The figure shows three views and two pictorial views of one solid part (mm, origin at its lowest corner). Answer the questions. A direction names the side the tool comes from. Round coordinates to 2 decimals unless told otherwise and drop trailing zeros. Order: outer loops, then holes, each group sorted by start corner. A loop starts at its lowest first (then second) coordinate and runs counter-clockwise, first axis right, second up. Notation, with made-up numbers: (4, 76.25) - (60, 76.25) arc R28 ccw to (60, 102.25) - close; hole circle Ø9 at (15.25, -18.5). An arc over 180 degrees is marked (long way). Use CSV: the item, a comma, the result in double quotes. Start each with the question number.
Item 1: Straight lines are drawn through the part: line 1 along Z through (x, y) = (62, 37); line 2 along X through (y, z) = (27.5, 6); line 3 along Z through (x, y) = (37.5, 33.5). For each, find the intervals that lie inside material, in ascending order. Write a range as [from, to].
Item 2: Find section D-D, the plane z = 26. Give the vertices of the cut face in (x, y).
Item 3: Find section A-A, the plane y = 20. Give the vertices of the cut face in (x, z), plus the area to 3 significant figures.
Item 4: Find section C-C, the plane x = 55. Give the vertices of the cut face in (y, z), plus the area to 3 significant figures.
Item 5: Flat-ended cylindrical pins translate along their axes: P1, Ø4.5, axis at x = 62, z = 46, coming from the -Y side; P2, Ø1.5, axis at x = 63, z = 6, coming from the +Y side; P3, Ø6, axis at x = 62, z = 6, coming from the -Y side. Find the tip coordinate at first contact, or state that the pin passes through.
Item 6: For the marked faces 1 and 2, determine the directions among +Z, -Z, +X, -X, +Y, -Y from which every point of the face is accessible in a straight line to the end or side of a thin tool.
Item 7: Find section B-B, the plane z = 46. Give the vertices of the cut face in (x, y).
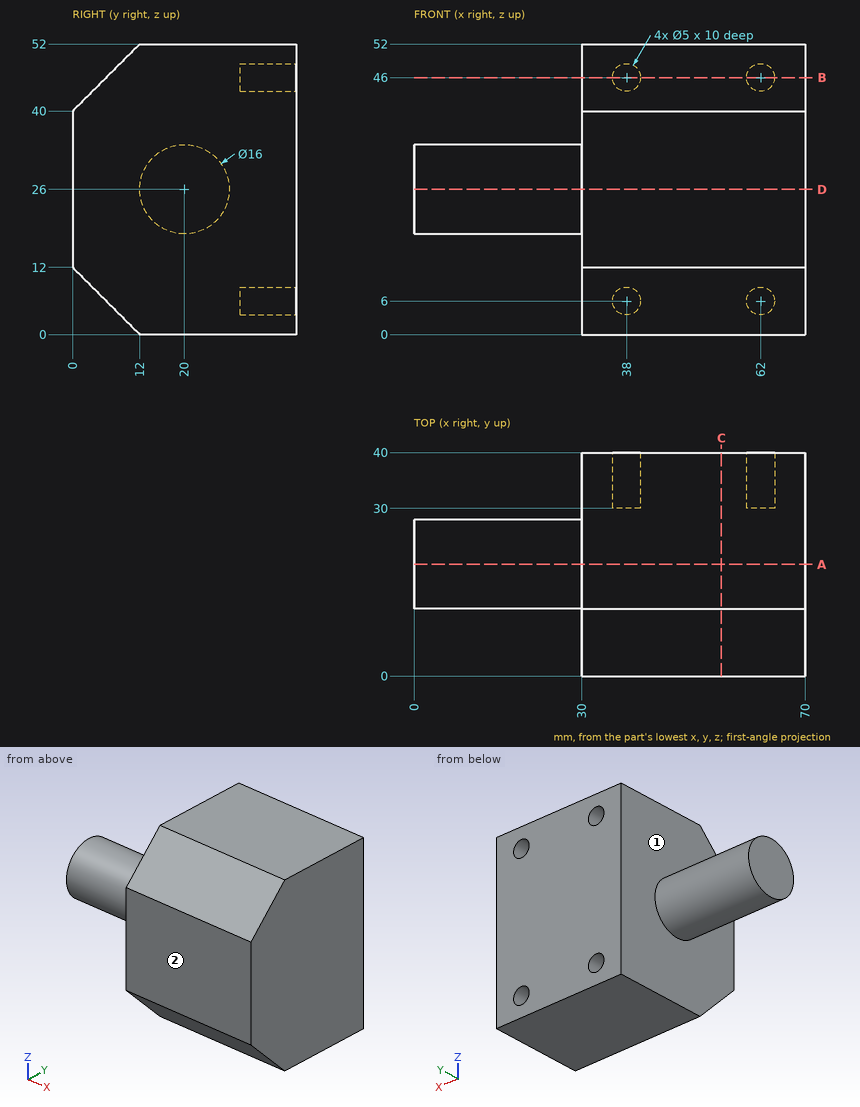
Worked out:
1,line 1,"z = [0, 3.5], [8.5, 43.5], [48.5, 52]"
1,line 2,"x = [30, 70]"
1,line 3,"z = [0, 3.55], [8.45, 43.55], [48.45, 52]"
2,outline,"(0, 12) - (30, 12) - (30, 0) - (70, 0) - (70, 40) - (30, 40) - (30, 28) - (0, 28) - close"
3,outline,"(0, 18) - (30, 18) - (30, 0) - (70, 0) - (70, 52) - (30, 52) - (30, 34) - (0, 34) - close"
3,area,"2,560 mm²"
4,outline,"(0, 12) - (12, 0) - (40, 0) - (40, 52) - (12, 52) - (0, 40) - close"
4,area,"1,940 mm²"
5,P1,"stops at y = 3.75"
5,P2,"stops at y = 30"
5,P3,"stops at y = 3"
6,face 1,"-X"
6,face 2,"+Z, -Z, +X, -X, -Y"
7,outline,"(30, 6) - (70, 6) - (70, 40) - (64.5, 40) - (64.5, 30) - (59.5, 30) - (59.5, 40) - (40.5, 40) - (40.5, 30) - (35.5, 30) - (35.5, 40) - (30, 40) - close"
